Build history of the part. All positions in model axes, mm. Face numbers are marked on the shaded views. A direction names the side the tool comes from. Coordinates: 2 decimals unless noted, no trailing zeros. Loops run counter-clockwise (first coordinate to the right, second up) from the corner with the lowest first, then second, coordinate; pieces in that order, holes last.
Item 1: Drill centre lines: line 1 along Y through (x, z) = (59, 94); line 2 along Y through (x, z) = (-30, 94); line 3 along X through (y, z) = (-30, 33.5). Where is each one in solid material? Low to high.
Item 2: Flat gauge pins, fed straight in: pin 1 (5 mm diameter, centred on y = 2, z = 79.5, fed in from -X); pin 2 (5 mm diameter, centred on x = -9.5, z = 24, fed in from +Y); pin 3 (10 mm diameter, centred on x = -50, z = 85.5, fed in from +Y). Where does each tip first touch, or does it go through?
Item 3: 3-axis set-ups, long thin cutter, end or side, ignore diameter. For the marked faces 4, 5 and 6: which of +Z, -Z, +X, -X, +Y, -Y reach the whole face in a straight line?
Item 4: Cut at A-A (x = 44). List the corners of the cut face in (y, z), and give its area (3 significant figures).
Item 5: Mould opens along Y. For the marked faces 1, 2 and 3 say: released by +Y, released by -Y, zero draft, split by the parting line, or undercut.
Item 6: Cut at B-B (y = 59). Count the separate pieces of the cut face and the enclosed holes in it, and give its area (3 significant figures).
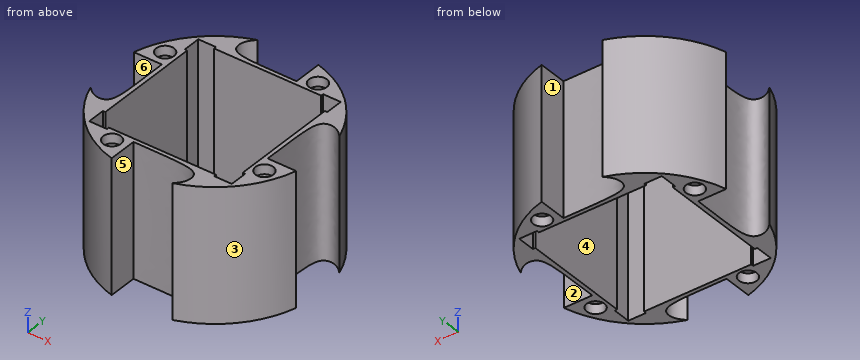
from build123d import *

# Parameters (mm, degrees)
BOSS_EXTRUDE3_OUTLINE_R = 3
BOSS_EXTRUDE3_DEPTH     = 97
SKETCH3_R               = 3
BOSS_EXTRUDE4_DEPTH     = 5
SKETCH3_3_R             = 6.5
CUT_EXTRUDE1_DEPTH      = 7
BOSS_EXTRUDE5_OUTLINE_R = 3
BOSS_EXTRUDE5_DEPTH     = 6
CUT_EXTRUDE2_DEPTH      = 6
SKETCH6_R               = 6.5
CUT_EXTRUDE5_DEPTH      = 7
CUT_EXTRUDE6_DEPTH      = 97
CUT_EXTRUDE9_DEPTH      = 97
SKETCH9_W               = 0.4
SKETCH9_H               = 1.8
SKETCH9_W_2             = 1.8
SKETCH9_H_2             = 0.4
BOSS_EXTRUDE6_DEPTH     = 97


# Read off the part's stored shape, not the designer's step: Boss-Extrude3, Boss-Extrude5, Cut-Extrude2
with BuildPart() as part:
    # Boss-Extrude3 outline → Boss-Extrude3 (new body)
    with BuildSketch(Plane.XY):
        with BuildLine():
            ThreePointArc((-24.28, 72.228260397), (-55.793380191, 51.899313356), (-73.793224621, 19))
            Line((-73.793224621, 19), (-53.359615493, 19))
            add(Edge.make_bspline(
                [(-72.206415586, -24.344887517), (-69.541086329, -27.040667073), (-67.428574969, -29.089162938), (-64.355831171, -30.241441862), (-60.963009895, -31.073643307), (-59.042545022, -30.561519341), (-56.673971678, -29.217193929), (-54.241382838, -27.488775543), (-53, -25.105954954), (-53, -17.37432721), (-53.359615493, 19)],
                knots=[0, 0, 0, 0, 0, 0, 0, 0, 0, 0, 0, 1, 1, 1, 1, 1, 1, 1, 1, 1, 1, 1], degree=10))
            ThreePointArc((-72.206415586, -24.344887517), (-51.874242853, -55.816690411), (-19, -73.793224621))
            Line((-19, -73.793224621), (-19, -53))
            add(Edge.make_bspline(
                [(24.344887517, -72.206415586), (27.040667073, -69.541086329), (29.089162938, -67.428574969), (30.241441862, -64.355831171), (31.073643307, -60.963009895), (30.561519341, -59.042545022), (29.217193929, -56.673971678), (27.488775543, -54.241382838), (25.105954954, -53), (17.37432721, -53), (-19, -53)],
                knots=[0, 0, 0, 0, 0, 0, 0, 0, 0, 0, 0, 1, 1, 1, 1, 1, 1, 1, 1, 1, 1, 1], degree=10))
            ThreePointArc((24.344887517, -72.206415586), (55.816690411, -51.874242853), (73.793224621, -19))
            Line((73.793224621, -19), (53, -19))
            add(Edge.make_bspline(
                [(72.227927536, 24.280990174), (69.541086329, 27.040667073), (67.428574969, 29.089162938), (64.355831171, 30.241441862), (60.963009895, 31.073643307), (59.042545022, 30.561519341), (56.673971678, 29.217193929), (54.241382838, 27.488775543), (53, 25.105954954), (53, 17.37432721), (53, -19)],
                knots=[0, 0, 0, 0, 0, 0, 0, 0, 0, 0, 0, 1, 1, 1, 1, 1, 1, 1, 1, 1, 1, 1], degree=10))
            ThreePointArc((72.227927536, 24.280990174), (51.89893092, 55.793735933), (19, 73.793224621))
            Line((19, 73.793224621), (19, 53))
            add(Edge.make_bspline(
                [(-24.28, 72.228260397), (-27.040667073, 69.541086329), (-29.089162938, 67.428574969), (-30.241441862, 64.355831171), (-31.073643307, 60.963009895), (-30.561519341, 59.042545022), (-29.217193929, 56.673971678), (-27.488775543, 54.241382838), (-25.105954954, 53), (-17.37432721, 53), (19, 53)],
                knots=[0, 0, 0, 0, 0, 0, 0, 0, 0, 0, 0, 1, 1, 1, 1, 1, 1, 1, 1, 1, 1, 1], degree=10))
        make_face()
        with Locations((-30, -59)):
            Circle(BOSS_EXTRUDE3_OUTLINE_R, mode=Mode.SUBTRACT)
        Polygon((-38.9, -51.6), (-51.6, -51.6), (-51.6, -38.9), (-50, -38.9), (-50, 38.9), (-51.6, 38.9), (-51.6, 51.6), (-38.9, 51.6), (-38.9, 50), (38.9, 50), (38.9, 51.6), (51.6, 51.6), (51.6, 38.9), (50, 38.9), (50, -38.9), (51.6, -38.9), (51.6, -51.6), (38.9, -51.6), (38.9, -50), (-38.9, -50), align=None, mode=Mode.SUBTRACT)
        with Locations((59, -30)):
            Circle(BOSS_EXTRUDE3_OUTLINE_R, mode=Mode.SUBTRACT)
        with Locations((-59.359615493, 30)):
            Circle(BOSS_EXTRUDE3_OUTLINE_R, mode=Mode.SUBTRACT)
        with Locations((30, 59)):
            Circle(BOSS_EXTRUDE3_OUTLINE_R, mode=Mode.SUBTRACT)
    extrude(amount=BOSS_EXTRUDE3_DEPTH)

    # Sketch3 → Boss-Extrude4 (add)
    with BuildSketch(Plane.XY.offset(97)):
        with Locations(Location((-59.359615493, 30, 0), (0, 0, 180))):
            Circle(SKETCH3_R)
    extrude(amount=BOSS_EXTRUDE4_DEPTH)


with BuildPart() as boss_extrude4_kept_piece:
    # of the separate pieces the step leaves, the one the design keeps (boss_extrude4_pieces_kept)
    add(part.part.solids().sort_by_distance((-24.28, 72.228260397, 0))[0])

    # Sketch3<3> → Cut-Extrude1 (cut)
    with BuildSketch(Plane.XY.offset(97)):
        with Locations((-59.359615493, 30)):
            Circle(SKETCH3_3_R)
        with Locations((30, 59)):
            Circle(SKETCH3_3_R)
        with Locations((59, -30)):
            Circle(SKETCH3_3_R)
        with Locations((-30, -59)):
            Circle(SKETCH3_3_R)
    extrude(amount=-CUT_EXTRUDE1_DEPTH, mode=Mode.SUBTRACT)

    # Boss-Extrude5 outline → Boss-Extrude5 (add)
    with BuildSketch(Plane.XY):
        with Locations((-59.359615493, 30)):
            Circle(BOSS_EXTRUDE5_OUTLINE_R)
    extrude(amount=BOSS_EXTRUDE5_DEPTH)

    # Cut-Extrude2 outline → Cut-Extrude2 (cut)
    with BuildSketch(Plane.XY):
        Polygon((-32.75, -54.236860279), (-35.5, -59), (-32.75, -63.763139721), (-27.25, -63.763139721), (-24.5, -59), (-27.25, -54.236860279), align=None)
        Polygon((59, -24.5), (54.236860279, -27.25), (54.236860279, -32.75), (59, -35.5), (63.763139721, -32.75), (63.763139721, -27.25), align=None)
        Polygon((-59.359615493, 35.5), (-64.122755214, 32.75), (-64.122755214, 27.25), (-59.359615493, 24.5), (-54.596475772, 27.25), (-54.596475772, 32.75), align=None)
        Polygon((32.75, 63.763139721), (27.25, 63.763139721), (24.5, 59), (27.25, 54.236860279), (32.75, 54.236860279), (35.5, 59), align=None)
    extrude(amount=CUT_EXTRUDE2_DEPTH, mode=Mode.SUBTRACT)

    # Sketch6 → Cut-Extrude5 (cut)
    with BuildSketch(Plane(origin=(0, 0, 0), x_dir=(-1, 0, 0), z_dir=(0, 0, -1))):
        with Locations(Location((-30, 59, 0), (0, 0, 180))):
            Circle(SKETCH6_R)
        with Locations(Location((59.359615493, 30, 0), (0, 0, 180))):
            Circle(SKETCH6_R)
        with Locations(Location((30, -59, 0), (0, 0, 180))):
            Circle(SKETCH6_R)
        with Locations(Location((-59, -30, 0), (0, 0, 180))):
            Circle(SKETCH6_R)
    extrude(amount=-CUT_EXTRUDE5_DEPTH, mode=Mode.SUBTRACT)

    # Sketch7 → Cut-Extrude6 (cut)
    with BuildSketch(Plane.XY.offset(97)):
        Polygon((-38.7, -51.8), (-51.8, -51.8), (-51.8, -38.7), (-50.2, -38.7), (-50.2, 38.7), (-51.8, 38.7), (-51.8, 51.8), (-38.7, 51.8), (-38.7, 50.2), (38.7, 50.2), (38.7, 51.8), (51.8, 51.8), (51.8, 38.7), (50.2, 38.7), (50.2, -38.7), (51.8, -38.7), (51.8, -51.8), (38.7, -51.8), (38.7, -50.2), (-38.7, -50.2), align=None)
        Polygon((-38.9, -51.6), (-51.6, -51.6), (-51.6, -38.9), (-50, -38.9), (-50, 38.9), (-51.6, 38.9), (-51.6, 51.6), (-38.9, 51.6), (-38.9, 50), (38.9, 50), (38.9, 51.6), (51.6, 51.6), (51.6, 38.9), (50, 38.9), (50, -38.9), (51.6, -38.9), (51.6, -51.6), (38.9, -51.6), (38.9, -50), (-38.9, -50), align=None, mode=Mode.SUBTRACT)
    extrude(amount=-CUT_EXTRUDE6_DEPTH, mode=Mode.SUBTRACT)

    # Sketch8 → Cut-Extrude9 (cut)
    with BuildSketch(Plane.XY.offset(97)):
        Polygon((-51.8, 38.7), (-51.8, 51.8), (-38.7, 51.8), (-38.7, 52), (-52, 52), (-52, 38.7), align=None)
        Polygon((-51.8, -38.7), (-51.8, -51.8), (-38.7, -51.8), (-38.7, -52), (-52, -52), (-52, -38.7), align=None)
        Polygon((51.8, -38.7), (51.8, -51.8), (38.7, -51.8), (38.7, -52), (52, -52), (52, -38.7), align=None)
        Polygon((51.8, 38.7), (51.8, 51.8), (38.7, 51.8), (38.7, 52), (52, 52), (52, 38.7), align=None)
    extrude(amount=-CUT_EXTRUDE9_DEPTH, mode=Mode.SUBTRACT)

    # Sketch9 → Boss-Extrude6 (add)
    with BuildSketch(Plane.XY.offset(97)):
        with Locations((-38.9, 51.1)):
            Rectangle(SKETCH9_W, SKETCH9_H)
        with Locations((-51.1, 38.9)):
            Rectangle(SKETCH9_W_2, SKETCH9_H_2)
        with Locations((38.9, 51.1)):
            Rectangle(SKETCH9_W, SKETCH9_H)
        with Locations((51.1, 38.9)):
            Rectangle(SKETCH9_W_2, SKETCH9_H_2)
        with Locations((51.1, -38.9)):
            Rectangle(SKETCH9_W_2, SKETCH9_H_2)
        with Locations((38.9, -51.1)):
            Rectangle(SKETCH9_W, SKETCH9_H)
        with Locations((-51.1, -38.9)):
            Rectangle(SKETCH9_W_2, SKETCH9_H_2)
        with Locations((-38.9, -51.1)):
            Rectangle(SKETCH9_W, SKETCH9_H)
    extrude(amount=-BOSS_EXTRUDE6_DEPTH)


solid = boss_extrude4_kept_piece.part
Filled sheet:
1. line 1: y = -48.22 to -36.5, -23.5 to -19, 29.41 to 48.22
1. line 2: y = -70.05 to -65.5, -52.5 to -50.2, 50.2 to 70.05
1. line 3: x = -70.05 to -50.2, 50.2 to 56, 62 to 70.05
2. pin 1: stops at x = -53.24
2. pin 2: stops at y = 53.27
2. pin 3: stops at y = 61.49
3. face 4: +Z, -Z
3. face 5: +Z, -Z, -Y
3. face 6: +Z, -Z, -X
4. outline: (-62.21, 0) - (-52, 0) - (-52, 97) - (-62.21, 97) - close; (52, 0) - (62.21, 0) - (62.21, 97) - (52, 97) - close
4. area: 1,980 mm2
5. face 1: zero draft
5. face 2: undercut
5. face 3: released by -Y
6. separate pieces: 3
6. enclosed holes: 0
6. area: 3,980 mm2
